```python
from build123d import *

# Parameters (mm, degrees)
F0_R     = 8
F1_DEPTH = 3
F2_DEPTH = 25


with BuildPart() as f1:
    # F0 (on Front) → F1 (new body)
    with BuildSketch(Plane.XZ):
        with BuildLine():
            Line((26.000001, 23.203813), (-33.999999, 23.203813))
            ThreePointArc((-33.999999, 23.203813), (-37.535533, 21.739347), (-38.999999, 18.203813))
            Line((-38.999999, 18.203813), (-38.999999, -23.796187))
            Line((-38.999999, -23.796187), (-20.999999, -23.796187))
            Line((-20.999999, -23.796187), (-20.999999, -26.796187))
            Line((-20.999999, -26.796187), (-12.999999, -26.796187))
            Line((-12.999999, -26.796187), (-12.999999, -23.796187))
            Line((-12.999999, -23.796187), (5.000001, -23.796187))
            Line((5.000001, -23.796187), (5.000001, -26.796187))
            Line((5.000001, -26.796187), (13.000001, -26.796187))
            Line((13.000001, -26.796187), (13.000001, -23.796187))
            Line((13.000001, -23.796187), (31.000001, -23.796187))
            Line((31.000001, -23.796187), (31.000001, 18.203813))
            ThreePointArc((31.000001, 18.203813), (29.535535, 21.739347), (26.000001, 23.203813))
        make_face()
        with Locations((-17, 0)):
            Circle(F0_R, mode=Mode.SUBTRACT)
        with Locations((9, 0)):
            Circle(F0_R, mode=Mode.SUBTRACT)
    extrude(amount=F1_DEPTH)


with BuildPart() as f2:
    # F0 (on Front) → F2 (new body)
    with BuildSketch(Plane.XZ):
        with BuildLine():
            Line((26.000001, 23.203813), (-33.999999, 23.203813))
            ThreePointArc((-33.999999, 23.203813), (-37.535533, 21.739347), (-38.999999, 18.203813))
            Line((-38.999999, 18.203813), (-38.999999, -23.796187))
            Line((-38.999999, -23.796187), (-20.999999, -23.796187))
            Line((-20.999999, -23.796187), (-20.999999, -26.796187))
            Line((-20.999999, -26.796187), (-12.999999, -26.796187))
            Line((-12.999999, -26.796187), (-12.999999, -23.796187))
            Line((-12.999999, -23.796187), (5.000001, -23.796187))
            Line((5.000001, -23.796187), (5.000001, -26.796187))
            Line((5.000001, -26.796187), (13.000001, -26.796187))
            Line((13.000001, -26.796187), (13.000001, -23.796187))
            Line((13.000001, -23.796187), (31.000001, -23.796187))
            Line((31.000001, -23.796187), (31.000001, 18.203813))
            ThreePointArc((31.000001, 18.203813), (29.535535, 21.739347), (26.000001, 23.203813))
        make_face()
        with Locations((-17, 0)):
            Circle(F0_R, mode=Mode.SUBTRACT)
        with Locations((9, 0)):
            Circle(F0_R, mode=Mode.SUBTRACT)
    extrude(amount=F2_DEPTH)


solid = f1.part
```
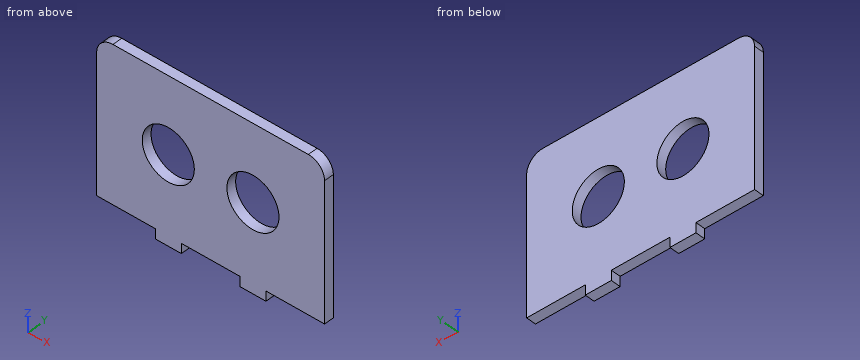
Work out the finished part from the listing and answer in its coordinate system (mm). Coordinates: 2 decimals unless noted, no trailing zeros. Loops run counter-clockwise (first coordinate to the right, second up) from the corner with the lowest first, then second, coordinate; pieces in that order, holes last.
1) Section A-A (z = 0) is taken. Give the vertices of the cut face in (x, y).
Results:
outline: (-39, -3) - (-25, -3) - (-25, 0) - (-39, 0) - close; (-9, -3) - (1, -3) - (1, 0) - (-9, 0) - close; (17, -3) - (31, -3) - (31, 0) - (17, 0) - close
2) Section D-D (x = -15) is taken. Give the vertices of the cut face in (y, z), plus the area to 3 significant figures.
Results:
outline: (-3, -26.8) - (0, -26.8) - (0, -7.75) - (-3, -7.75) - close; (-3, 7.75) - (0, 7.75) - (0, 23.2) - (-3, 23.2) - close
area: 104 mm2
3) Flat-ended cylindrical pins translate along their axes: pin 1 (1 mm diameter, centred on x = 4, y = -1, fed in from -Z); pin 2 (14.5 mm diameter, centred on x = 9, z = 0, fed in from +Y); pin 3 (0.9 mm diameter, centred on y = -2, z = -25.5, fed in from -X); pin 4 (1.5 mm diameter, centred on y = -2, z = -25, fed in from +X). Find the tip coordinate at first contact, or state that the pin passes through.
Results:
pin 1: stops at z = -23.8
pin 2: passes through
pin 3: stops at x = -21
pin 4: stops at x = 13
4) Section C-C (x = 9) is taken. Give the vertices of the cut face in (y, z), plus the area to 3 significant figures.
Results:
outline: (-3, -26.8) - (0, -26.8) - (0, -8) - (-3, -8) - close; (-3, 8) - (0, 8) - (0, 23.2) - (-3, 23.2) - close
area: 102 mm2
5) Section B-B (y = -2.45) is taken. Give the vertices of the cut face in (x, z), plus the area to 3 significant figures.
Results:
outline: (-39, -23.8) - (-21, -23.8) - (-21, -26.8) - (-13, -26.8) - (-13, -23.8) - (5, -23.8) - (5, -26.8) - (13, -26.8) - (13, -23.8) - (31, -23.8) - (31, 18.2) arc R5 ccw to (26, 23.2) - (-34, 23.2) arc R5 ccw to (-39, 18.2) - close; hole circle Ø16 at (-17, 0); hole circle Ø16 at (9, 0)
area: 2,930 mm2
6) Consider probe 1 along X at (y, z) = (-2.45, 0.5); probe 2 along Z at (x, y) = (-17, -1.65); probe 3 along X at (y, z) = (-0.2, -6.5). Determine where each line is inside the solid, lowest interval first.
Results:
probe 1: x = -39 to -24.98, -9.02 to 1.02, 16.98 to 31
probe 2: z = -26.8 to -8, 8 to 23.2
probe 3: x = -39 to -21.66, -12.34 to 4.34, 13.66 to 31
